Geometry: see drawing. Coordinates: mm, zero at the bounding-box minimum. Coordinates: 2 decimals unless noted, no trailing zeros. Write each loop counter-clockwise with the first axis right and the second up, starting at its lowest first coordinate (ties: lowest second). Pieces come first, ordered by that corner, then holes. Notation, with made-up numbers: M -24.5,8.25 L -2.5,8.25 A14 cw -2.5,12.25 Z; hole C 61.5,44 d3. An arc over 180 degrees is marked long. Answer as CSV lines item,"result". Start each with the question number.
1. Section B-B on z = 23.5. Return the cut outline in (x, y), plus the area to 3 significant figures.
2. Line query: probe 1 along X at (y, z) = (1.4, 29); probe 2 along Z at (x, y) = (15.5, 2.5); probe 3 along Z at (x, y) = (19, 2.35). Output: solid intervals per line, ascending. Write a range as [from, to].
3. Section A-A on x = 9.5. Return the cut outline in (y, z).
4. Section C-C on y = 1.5. Return the cut outline in (x, z), plus the area to 3 significant figures.
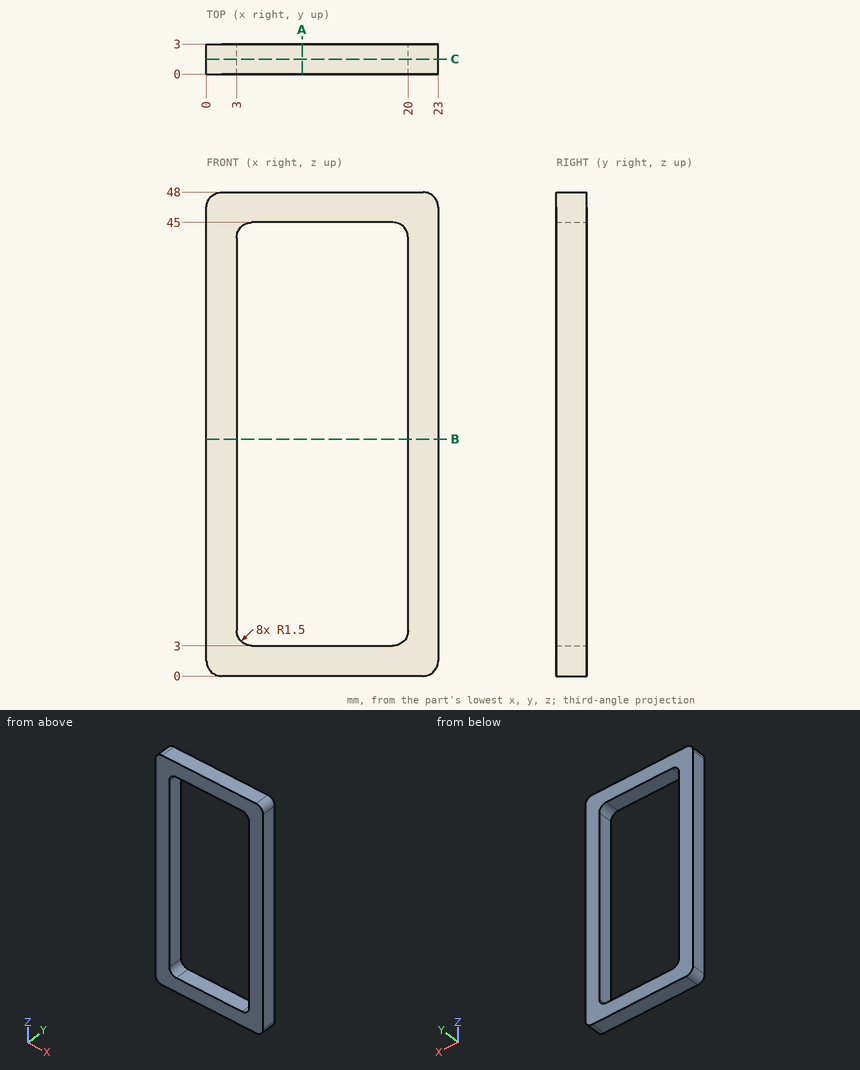
Values:
1,outline,"M 0,0 L 3,0 L 3,3 L 0,3 Z; M 20,0 L 23,0 L 23,3 L 20,3 Z"
1,area,"18.0 mm²"
2,probe 1,"[0, 3], [20, 23]"
2,probe 2,"[0, 3], [45, 48]"
2,probe 3,"[0, 3.09], [44.91, 48]"
3,outline,"M 0,0 L 3,0 L 3,3 L 0,3 Z; M 0,45 L 3,45 L 3,48 L 0,48 Z"
4,outline,"M 0,1.5 A1.5 ccw 1.5,0 L 21.5,0 A1.5 ccw 23,1.5 L 23,46.5 A1.5 ccw 21.5,48 L 1.5,48 A1.5 ccw 0,46.5 Z; hole M 3,4.5 A1.5 ccw 4.5,3 L 18.5,3 A1.5 ccw 20,4.5 L 20,43.5 A1.5 ccw 18.5,45 L 4.5,45 A1.5 ccw 3,43.5 Z"
4,area,"390 mm²"
